The figure shows three views and two pictorial views of one solid part (mm, origin at its lowest corner). Answer the questions. A direction names the side the tool comes from. Round coordinates to 2 decimals unless told otherwise and drop trailing zeros. Order: outer loops, then holes, each group sorted by start corner. A loop starts at its lowest first (then second) coordinate and runs counter-clockwise, first axis right, second up.
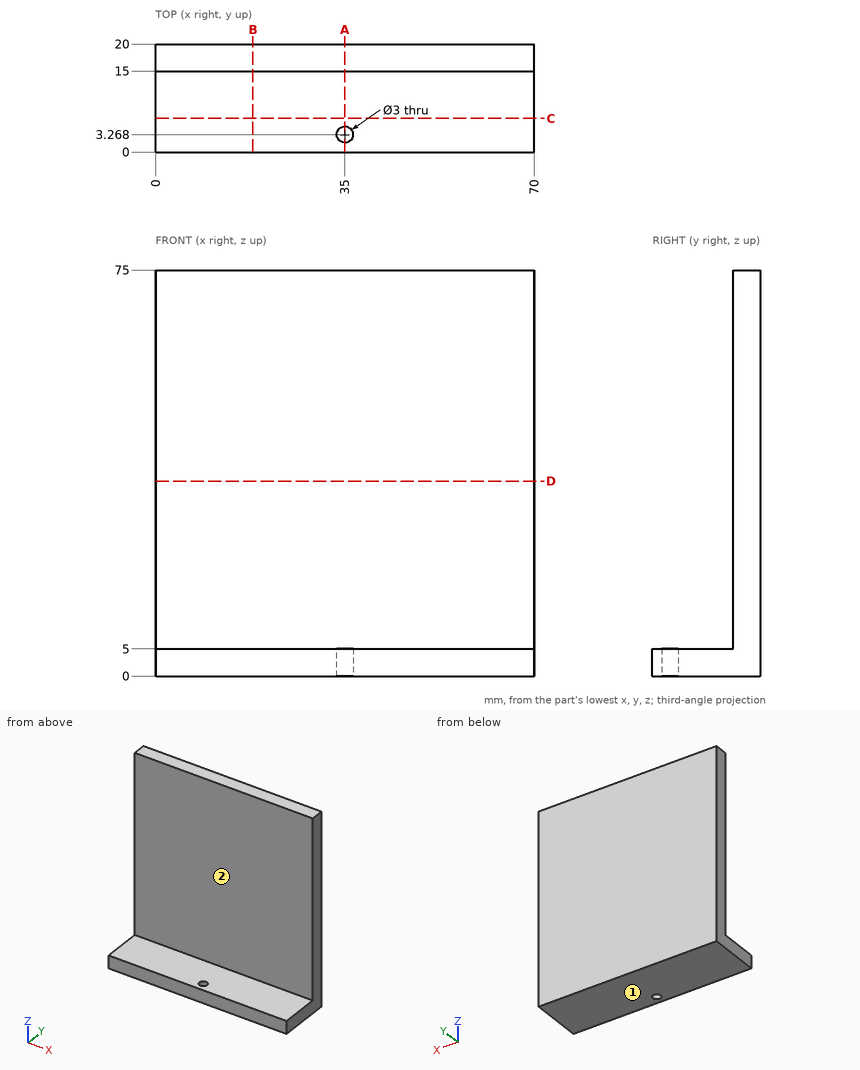
Item 1: A tool of negligible diameter and unlimited length cuts with its end or side. For the marked faces 1 and 2, from which of +Z, -Z, +X, -X, +Y, -Y can it reach the whole face along a straight path? Write none if from no direction.
Item 2: Find section C-C (y = 6.25). Write down the section's boundary in (x, z).
Item 3: Find section D-D (z = 36). Write down the section's boundary in (x, y), plus the area to 3 significant figures.
Item 4: Find section A-A (x = 35). Write down the section's boundary in (y, z).
Item 5: Given pin 1 (12 mm diameter, centred on x = 53.5, z = 44.5, fed in from -Y); pin 2 (10 mm diameter, centred on x = 31.5, y = 6.5, fed in from +Z), each flat-ended and moving along its own axis, determine where each tip first touches the part or whether it passes through.
Item 6: Find the intervals of material crossed by line 1 along Y through (x, z) = (35, 3.8); line 2 along Z through (x, y) = (33.5, 2); line 3 along Y through (x, z) = (10.5, 62.5), in increasing order.
Item 7: Find section B-B (x = 18). Write down the section's boundary in (y, z), plus the area to 3 significant figures.
Model answer:
1. face 1: -Z, +X, -X, +Y, -Y
1. face 2: +Z, +X, -X, -Y
2. outline: (0, 0) - (70, 0) - (70, 5) - (0, 5) - close
3. outline: (0, 15) - (70, 15) - (70, 20) - (0, 20) - close
3. area: 350 mm2
4. outline: (0, 0) - (1.77, 0) - (1.77, 5) - (0, 5) - close; (4.77, 0) - (20, 0) - (20, 75) - (15, 75) - (15, 5) - (4.77, 5) - close
5. pin 1: stops at y = 15
5. pin 2: stops at z = 5
6. line 1: y = 0 to 1.77, 4.77 to 20
6. line 2: z = 0 to 5
6. line 3: y = 15 to 20
7. outline: (0, 0) - (20, 0) - (20, 75) - (15, 75) - (15, 5) - (0, 5) - close
7. area: 450 mm2
